For this review, take the finished solid that the model builds, in its own axes (mm). A direction names the side the tool comes from. Give positions to 0.01 mm unless a question says otherwise; leave off trailing zeros. Write each loop counter-clockwise with the first axis right and the second up, starting at its lowest first coordinate (ties: lowest second). Pieces come first, ordered by that corner, then holes. Notation, with made-up numbers: M -30,-15 L -21,-15 A4 ccw -21,-8 Z; hole C -2,-19.75 d10. An arc over 180 degrees is marked long. One line per item, written item: value. Start each with the question number.
Item 1: Consider section A-A, the plane z = 0. Write out the cut boundary in (x, y).
Item 2: Mouldability with a two-part tool opening along Z and no side actions: class faces 3 (the face through (-10, 40, 0)), 4 (the face through (0, 40, -11)), 5 (the face through (-11.497, 40.384, 0.253)) as released by +Z, released by -Z, zero draft, split by the parting line, or undercut.
Item 3: To check wall thickness, follow probe 1 along Y at (x, z) = (-7.25, 6.25); probe 2 along Z at (x, y) = (-8.25, 69); probe 3 along Z at (x, y) = (-5, 10). State the ranges of each line that lie inside material, in increasing order.
Item 4: Consider section B-B, the plane x = -1.25. Write out the cut boundary in (y, z), and give its area (3 significant figures).
Item 5: Consider section D-D, the plane y = 15. Write out the cut boundary in (x, z).
Item 6: Consider section C-C, the plane x = -8.5. Write out the cut boundary in (y, z).
Item 7: Clearance check with flat-ended pins moving along their axes: pin 1 Ø6 at (y, z) = (12, -8.5) entering from -X; pin 2 Ø1.5 at (y, z) = (43, -6.5) entering from +X; pin 3 Ø5 at (x, y) = (-5.5, 43) entering from -Z. State where each tip first meets the part, or that it passes through.
Item 8: Tool access review of faces 1 (the face through (-8, 82, -1)), 2 (the face through (-7.75, -1.52, 0.17)): name each direction out of +Z, -Z, +X, -X, +Y, -Y from which nothing blocks a thin tool from reaching the whole face with its end or side.
Autodesk Inventor part; units mm, degrees
ref_plane "YZ Plane" through (0, 0, 0) normal (1, 0, 0) x (0, 1, 0)
ref_plane "XZ Plane" through (0, 0, 0) normal (0, 1, 0) x (-1, 0, 0)
ref_plane "XY Plane" through (0, 0, 0) normal (0, 0, 1) x (1, 0, 0)
sketch "草圖1" plane through (0, 0, 0) normal (0, 1, 0) x (-1, 0, 0)
  arc A0 (0, -10) -> (0, 10) centre (0, 0) ccw
  arc A1 (0, -11.5) -> (0, 11.5) centre (0, 0) ccw
  line L0 (0, 11.5) -> (0, 10)
  line L1 (0, -10) -> (0, -11.5)
  dimension "d0" = 20
  dimension "d1" = 23
extrude "擠出1" add sketch "草圖1" along normal blind 41
sketch "草圖2" plane through (0, 41, 0) normal (0, 1, 0) x (1, 0, 0)
  line L0 (0, -11.5) -> (0, -10)
  arc A0 (0, 11.5) -> (0, -11.5) centre (0, 0) ccw
  line L1 (0, 10) -> (0, 11.5)
  line L2 (0, -10) -> (0, 10)
extrude "擠出2" add sketch "草圖2" along normal blind 3
sketch "草圖3" plane through (0, 44, 0) normal (0, 1, 0) x (1, 0, 0)
  arc A0 (0, 7.75) -> (0, -7.75) centre (0, 0) ccw
  line L0 (0, -10) -> (0, 10)
  line L1 (0, -7.75) -> (0, 7.75)
  dimension "d7" = 15.5
extrude "擠出3" cut sketch "草圖3" against normal up to next
sketch "草圖5" plane through (0, 0, 0) normal (0, -1, 0) x (1, 0, 0)
  arc A0 (0, 10) -> (0, -10) centre (0, 0) ccw
  line L0 (0, 10) -> (0, 11.5)
  arc A1 (0, 11.5) -> (0, -11.5) centre (0, 0) ccw
  line L1 (0, -11.5) -> (0, -10)
  line L2 (0, 11.5) -> (0, -11.5)
extrude "擠出4" add sketch "草圖5" along normal blind 3
sketch "草圖7" plane through (0, -3, 0) normal (0, -1, 0) x (1, 0, 0)
  arc A0 (0, 7.75) -> (0, -7.75) centre (0, 0) ccw
  line L0 (0, -11.5) -> (0, 11.5)
  line L1 (0, -7.75) -> (0, 7.75)
  dimension "d13" = 15.5
extrude "擠出5" cut sketch "草圖7" against normal up to next
sketch "草圖8" plane through (0, 44, 0) normal (0, 1, 0) x (1, 0, 0)
  arc A0 (0, 11.5) -> (0, -11.5) centre (0, 0) ccw
  arc A1 (0, 10) -> (0, -10) centre (0, 0) ccw
  line L0 (0, 7.75) -> (0, 11.5)
  line L1 (0, 11.5) -> (0, 10)
  line L2 (0, -10) -> (0, -11.5)
extrude "擠出6" add sketch "草圖8" along normal blind 38
sketch "草圖9" plane through (0, 82, 0) normal (0, 1, 0) x (1, 0, 0)
  arc A0 (0, 11.5) -> (0, -11.5) centre (0, 0) ccw
  arc A1 (0, 7.75) -> (0, -7.75) centre (0, 0) ccw
  line L0 (0, 11.5) -> (0, 7.75)
  line L1 (0, -7.75) -> (0, -11.5)
extrude "擠出7" add sketch "草圖9" along normal blind 3
sketch "草圖10" plane through (0, 44, 0) normal (0, 1, 0) x (1, 0, 0)
  arc A0 (0, 10) -> (0, -10) centre (0, 0) ccw
  line L0 (0, -10) -> (0, -7.75)
  arc A1 (0, 7.75) -> (0, -7.75) centre (0, 0) ccw
  line L1 (0, 7.75) -> (0, 10)
extrude "擠出8" cut sketch "草圖10" against normal blind 3
sketch "Sketch11" plane through (0, 0, 0) normal (0, 0, 1) x (1, 0, 0)
  line L0 (0, 85) -> (-11.5, 85)
  line L1 (-11.5, -3) -> (0, -3)
  point P0 (0, 0)
  dimension "d22" = 88
properties part number "蓋子"
Model answer:
1. outline: M -11.5,-3 L -7.75,-3 L -7.75,0 L -10,0 L -10,82 L -7.75,82 L -7.75,85 L -11.5,85 Z
2. face 3: undercut
2. face 4: zero draft
2. face 5: split by the parting line
3. probe 1: y = -3 to 0, 82 to 85
3. probe 2: z = -8.01 to -5.65, 5.65 to 8.01
3. probe 3: z = -10.36 to -8.66, 8.66 to 10.36
4. outline: M -3,-11.43 L 85,-11.43 L 85,-7.65 L 82,-7.65 L 82,-9.92 L 0,-9.92 L 0,-7.65 L -3,-7.65 Z; M -3,7.65 L 0,7.65 L 0,9.92 L 82,9.92 L 82,7.65 L 85,7.65 L 85,11.43 L -3,11.43 Z
4. area: 293 mm2
5. outline: M 0,-11.5 L 0,-10 A10 cw 0,10 L 0,11.5 A11.5 ccw Z
6. outline: M -3,-7.75 L 85,-7.75 L 85,7.75 L -3,7.75 Z; hole M 0,-5.27 L 82,-5.27 L 82,5.27 L 0,5.27 Z
7. pin 1: stops at x = -10.1
7. pin 2: stops at x = -6.89
7. pin 3: stops at z = -11.1
8. face 1: +X
8. face 2: +X, +Y, -Y
